from build123d import *

# Parameters (mm, degrees)
SKETCH_1_W          = 330
SKETCH_1_H          = 330
EXTRUDE_1_DEPTH     = 5
SKETCH_2_R          = 1.6
SKETCH_2_R_2        = 1.602203763
CUT_EXTRUDE_1_DEPTH = 234.39880034
SKETCH_3_W          = 220
SKETCH_3_H          = 20
CUT_EXTRUDE_2_DEPTH = 234.39880034
SKETCH_4_W          = 20
SKETCH_4_H          = 220
CUT_EXTRUDE_3_DEPTH = 234.39880034
SKETCH_7_W          = 220
SKETCH_7_H          = 20
CUT_EXTRUDE_4_DEPTH = 234.39880034
SKETCH_9_W          = 239.54111937
SKETCH_9_H          = 233.56752537
EXTRUDE_2_DEPTH     = 5


with BuildPart() as part:
    # 草图1 → 凸台-拉伸1 (new body)
    with BuildSketch(Plane(origin=(0, 0, 0), x_dir=(1, 0, 0), z_dir=(0, 1, 0))):
        Rectangle(SKETCH_1_W, SKETCH_1_H)
    extrude(amount=EXTRUDE_1_DEPTH)

    # 草图2 → 切除-拉伸1 (cut, through all)
    with BuildSketch(Plane(origin=(0, 5, 0), x_dir=(1, 0, 0), z_dir=(0, 1, 0))):
        with Locations(Location((-159.5, 159, 0), (0, 0, 270))):
            Circle(SKETCH_2_R)
        with Locations(Location((-128.5, 159, 0), (0, 0, 270))):
            Circle(SKETCH_2_R)
        with Locations(Location((-159.5, 128, 0), (0, 0, 270))):
            Circle(SKETCH_2_R_2)
        with Locations(Location((-128.5, 128, 0), (0, 0, 270))):
            Circle(SKETCH_2_R)
        with Locations(Location((128.5, 159, 0), (0, 0, 270))):
            Circle(SKETCH_2_R)
        with Locations(Location((159.5, 159, 0), (0, 0, 270))):
            Circle(SKETCH_2_R)
        with Locations(Location((128.5, 128, 0), (0, 0, 270))):
            Circle(SKETCH_2_R)
        with Locations(Location((159.5, 128, 0), (0, 0, 270))):
            Circle(SKETCH_2_R)
        with Locations(Location((128.5, -128, 0), (0, 0, 270))):
            Circle(SKETCH_2_R)
        with Locations(Location((159.5, -128, 0), (0, 0, 270))):
            Circle(SKETCH_2_R)
        with Locations(Location((159.5, -159, 0), (0, 0, 270))):
            Circle(SKETCH_2_R)
        with Locations(Location((128.5, -159, 0), (0, 0, 270))):
            Circle(SKETCH_2_R)
        with Locations(Location((-128.5, -159, 0), (0, 0, 270))):
            Circle(SKETCH_2_R)
        with Locations(Location((-159.5, -159, 0), (0, 0, 270))):
            Circle(SKETCH_2_R)
        with Locations(Location((-159.5, -128, 0), (0, 0, 270))):
            Circle(SKETCH_2_R)
        with Locations(Location((-128.5, -128, 0), (0, 0, 270))):
            Circle(SKETCH_2_R)
    extrude(amount=-CUT_EXTRUDE_1_DEPTH, mode=Mode.SUBTRACT)

    # 草图3 → 切除-拉伸2 (cut, through all)
    with BuildSketch(Plane(origin=(0, 5, 0), x_dir=(1, 0, 0), z_dir=(0, 1, 0))):
        with Locations((0, 100)):
            Rectangle(SKETCH_3_W, SKETCH_3_H)
        with Locations((0, 50)):
            Rectangle(SKETCH_3_W, SKETCH_3_H)
        Rectangle(SKETCH_3_W, SKETCH_3_H)
        with Locations((0, -50)):
            Rectangle(SKETCH_3_W, SKETCH_3_H)
        with Locations((0, -100)):
            Rectangle(SKETCH_3_W, SKETCH_3_H)
    extrude(amount=-CUT_EXTRUDE_2_DEPTH, mode=Mode.SUBTRACT)

    # 草图4 → 切除-拉伸3 (cut, through all)
    with BuildSketch(Plane(origin=(0, 5, 0), x_dir=(1, 0, 0), z_dir=(0, 1, 0))):
        with Locations((-140, 0)):
            Rectangle(SKETCH_4_W, SKETCH_4_H)
        with Locations((140, 0)):
            Rectangle(SKETCH_4_W, SKETCH_4_H)
    extrude(amount=-CUT_EXTRUDE_3_DEPTH, mode=Mode.SUBTRACT)

    # 草图7 → 切除-拉伸4 (cut, through all)
    with BuildSketch(Plane(origin=(0, 5, 0), x_dir=(1, 0, 0), z_dir=(0, 1, 0))):
        with Locations((0, 140)):
            Rectangle(SKETCH_7_W, SKETCH_7_H)
        with Locations((0, -140)):
            Rectangle(SKETCH_7_W, SKETCH_7_H)
    extrude(amount=-CUT_EXTRUDE_4_DEPTH, mode=Mode.SUBTRACT)

    # 草图9 → 凸台-拉伸2 (add)
    with BuildSketch(Plane(origin=(0, 5, 0), x_dir=(1, 0, 0), z_dir=(0, 1, 0))):
        with Locations((2.0907579, 0.2986797)):
            Rectangle(SKETCH_9_W, SKETCH_9_H)
    extrude(amount=-EXTRUDE_2_DEPTH)


solid = part.part
Source: CAD feature listing. Evaluate the final solid. Frame: model axes, mm. Give positions to 0.01 mm unless a question says otherwise; leave off trailing zeros. Write each loop counter-clockwise with the first axis right and the second up, starting at its lowest first coordinate (ties: lowest second). Pieces come first, ordered by that corner, then holes. Notation, with made-up numbers: (-25, 15.25) -> (30, 15.25) arc R22 ccw to (30, 48.25) -> close; hole circle Ø4 at (6, -9.5). An arc over 180 degrees is marked (long way). Return JSON: item names as keys, results as strings. Group by question number.
1. Section A-A, the plane z = 52.5. Output: boundary loops of the cut face in (x, y).
2. Section C-C, the plane y = 0.95. Count the separate pieces of the cut face and the enclosed holes in it, then the cut area to 3 significant figures.
3. Section B-B, the plane x = -12.5. Output: boundary loops of the cut face in (y, z).
4. Material intervals for line 1 (X direction, y = 2.2, z = -128); line 2 (Z direction, x = -94.5, y = 3.65), sorted ascending. Write a range as from..to.
5. Pin query (flat end, axial travel): pin 1 Ø8 at (x, z) = (93, 51) entering from -Y. Return the tip coordinate at first contact, or that it passes through.
Determined:
{
 "1": {"outline": "(-165, 0) -> (-150, 0) -> (-150, 5) -> (-165, 5) -> close; (-130, 0) -> (130, 0) -> (130, 5) -> (-130, 5) -> close; (150, 0) -> (165, 0) -> (165, 5) -> (150, 5) -> close"},
 "2": {"separate pieces": "1", "enclosed holes": "20", "area": "91,200 mm2"},
 "3": {"outline": "(0, -165) -> (5, -165) -> (5, -150) -> (0, -150) -> close; (0, -130) -> (5, -130) -> (5, 130) -> (0, 130) -> close; (0, 150) -> (5, 150) -> (5, 165) -> (0, 165) -> close"},
 "4": {"line 1": "x = -165..-161.1, -157.9..-130.1, -126.9..126.9, 130.1..157.9, 161.1..165", "line 2": "z = -165..-150, -130..130, 150..165"},
 "5": {"pin 1": "stops at y = 0"}
}
